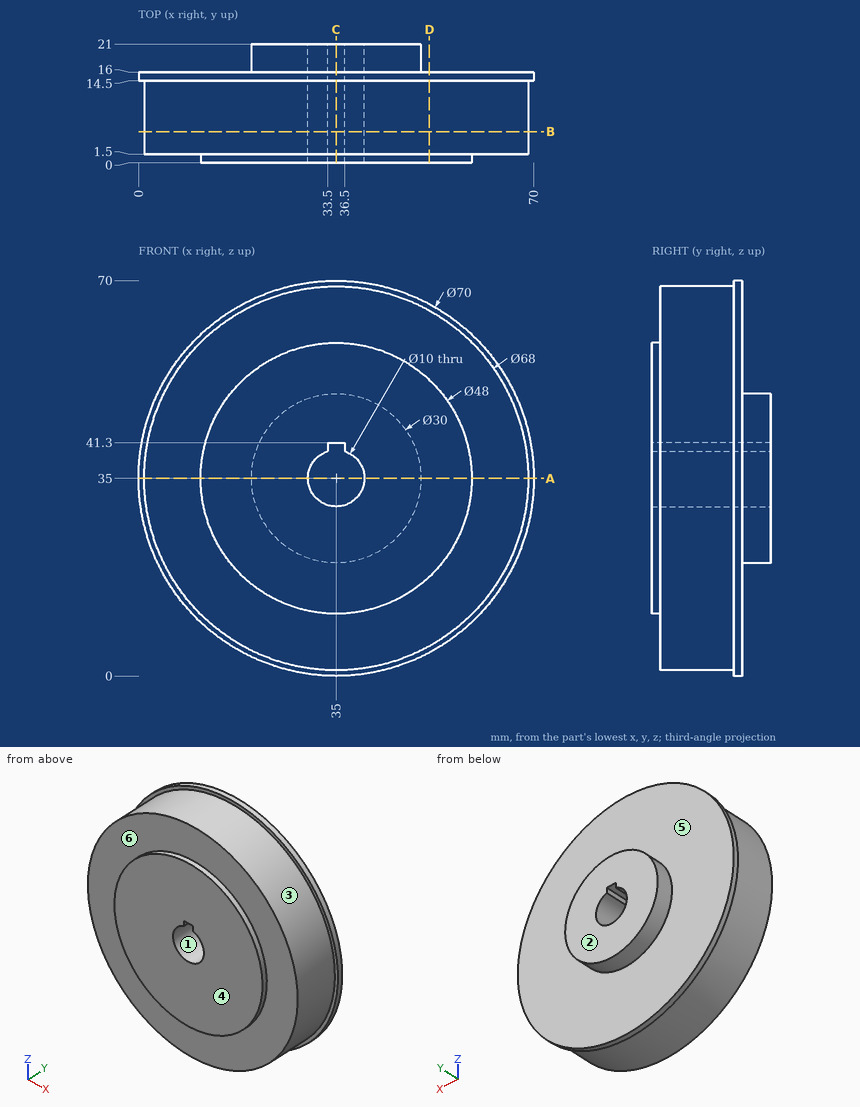
For this review, use the dimensioned drawing (mm, ordinates from the lowest corner) and the shaded views. A direction names the side the tool comes from. Coordinates: 2 decimals unless noted, no trailing zeros. Write each loop counter-clockwise with the first axis right and the second up, starting at its lowest first coordinate (ties: lowest second). Pieces come first, ordered by that corner, then holes. Notation, with made-up numbers: (77.5, 3) - (96.5, 3) arc R14 ccw to (96.5, 13) - close; hole circle Ø5 at (11, 56.25). An arc over 180 degrees is marked (long way). Answer in a Markdown table with one row per item. Add a question column.
Q1. Consider section B-B on y = 5.5. Give the boundary of the cut face in (x, z).
Q2. Consider section C-C on x = 35. Give the boundary of the cut face in (y, z), then the cut area to 3 significant figures.
Q3. For the marked faces 4, 5 and 6, list the 3-axis set-ups (+Z, -Z, +X, -X, +Y, -Y) from which the entire face can be reached by the end or side of a thin tool; tool diameter is ignored.
Q4. Clearance check with flat-ended pins moving along their axes: pin 1 (6 mm diameter, centred on x = 42.5, y = 12, fed in from -Z); pin 2 (12 mm diameter, centred on x = 33.5, y = 3, fed in from -Z); pin 3 (10 mm diameter, centred on x = 22, y = 12, fed in from +Z). State where each tip first meets the part, or that it passes through.
Q5. Consider section A-A on z = 35. Give the boundary of the cut face in (x, y).
Q6. Consider section D-D on x = 51.5. Give the boundary of the cut face in (y, z), then the cut area to 3 significant figures.
Q7. To check wall thickness, follow line 1 along X through (y, z) = (2.25, 4.5); line 2 along Y through (x, z) = (47, 52); line 3 along Y through (x, z) = (23.5, 60.5). State the ranges of each line that lie inside material, in increasing order. Write a range as from..to.
Q8. Draft analysis for pull direction X (two halves, no side actions). For the marked faces 1, 2 and 3, state which applies: +X half, -X half, draft (parallel to the pull), parting line (faces both ways), or undercut.
Answers below:
| question | item | result |
|---|---|---|
| 1 | outline | circle Ø68 at (35, 35); hole (33.5, 39.77) arc R5 ccw (long way) to (36.5, 39.77) - (36.5, 41.3) - (33.5, 41.3) - close |
| 2 | outline | (0, 11) - (1.5, 11) - (1.5, 1) - (14.5, 1) - (14.5, 0) - (16, 0) - (16, 20) - (21, 20) - (21, 30) - (0, 30) - close; (0, 41.3) - (21, 41.3) - (21, 50) - (16, 50) - (16, 70) - (14.5, 70) - (14.5, 69) - (1.5, 69) - (1.5, 59) - (0, 59) - close |
| 2 | area | 974 mm² |
| 3 | face 4 | +Z, -Z, +X, -X, -Y |
| 3 | face 5 | +Y |
| 3 | face 6 | -Y |
| 4 | pin 1 | z = 0.49 |
| 4 | pin 2 | z = 1 |
| 4 | pin 3 | z = 68.91 |
| 5 | outline | (0, 14.5) - (1, 14.5) - (1, 1.5) - (11, 1.5) - (11, 0) - (30, 0) - (30, 21) - (20, 21) - (20, 16) - (0, 16) - close; (40, 0) - (59, 0) - (59, 1.5) - (69, 1.5) - (69, 14.5) - (70, 14.5) - (70, 16) - (50, 16) - (50, 21) - (40, 21) - close |
| 6 | outline | (0, 17.57) - (1.5, 17.57) - (1.5, 5.27) - (14.5, 5.27) - (14.5, 4.13) - (16, 4.13) - (16, 65.87) - (14.5, 65.87) - (14.5, 64.73) - (1.5, 64.73) - (1.5, 52.43) - (0, 52.43) - close |
| 6 | area | 918 mm² |
| 7 | line 1 | 19.98..50.02 |
| 7 | line 2 | 0..16 |
| 7 | line 3 | 1.5..16 |
| 8 | face 1 | undercut |
| 8 | face 2 | draft |
| 8 | face 3 | parting line |
